Read the model definition and answer for the solid it produces. Units are mm, in the model's axes. Face numbers are marked on the shaded views. Give positions to 0.01 mm unless a question says otherwise; leave off trailing zeros. Write each loop counter-clockwise with the first axis right and the second up, starting at its lowest first coordinate (ties: lowest second). Pieces come first, ordered by that corner, then holes. Notation, with made-up numbers: (26.5, 51.25) -> (85.5, 51.25) arc R10 cw to (85.5, 69.25) -> close; hole circle Ø2 at (81, 3.25). An arc over 180 degrees is marked (long way). Use a Markdown table: item, result.
from build123d import *

# Parameters (mm, degrees)
CROQUIS1_R              = 105
CROQUIS1_R_2            = 95
SALIENTE_EXTRUIR1_DEPTH = 180
CROQUIS2_R              = 101.5
SALIENTE_EXTRUIR2_DEPTH = 20
REDONDEO1_R             = 15


with BuildPart() as part:
    # Croquis1 → Saliente-Extruir1 (new body)
    with BuildSketch(Plane.XY):
        with Locations(Location((0, 0, 0), (0, 0, 180))):
            Circle(CROQUIS1_R)
        with Locations(Location((0, 0, 0), (0, 0, 180))):
            Circle(CROQUIS1_R_2, mode=Mode.SUBTRACT)
    extrude(amount=SALIENTE_EXTRUIR1_DEPTH)

    # Croquis2 → Saliente-Extruir2 (add)
    with BuildSketch(Plane.XY.offset(180)):
        Circle(CROQUIS2_R)
    extrude(amount=-SALIENTE_EXTRUIR2_DEPTH)

    # Redondeo1
    redondeo1_edges = [part.edges().sort_by_distance(p)[0] for p in [
        (105, 0, 180),
    ]]
    fillet(redondeo1_edges, radius=REDONDEO1_R)


solid = part.part
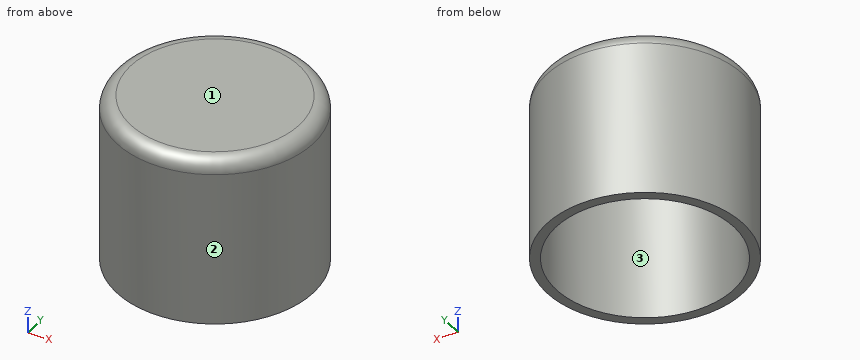
Item 1: For a pull along Y with two mould halves and no side action, classify the marked faces 1, 2 and 3 as +Y half, -Y half, draft (parallel to the pull), parting line (faces both ways), or undercut.
Return value:
| item | result |
|---|---|
| face 1 | draft |
| face 2 | parting line |
| face 3 | undercut |
Item 2: A cutting plane is placed at A-A (x = 0). Give the vertices of the cut face in (y, z), then the cut area to 3 significant figures.
Return value:
| item | result |
|---|---|
| outline | (-105, 0) -> (-95, 0) -> (-95, 160) -> (95, 160) -> (95, 0) -> (105, 0) -> (105, 165) arc R15 ccw to (90, 180) -> (-90, 180) arc R15 ccw to (-105, 165) -> close |
| area | 7,300 mm^2 |
Item 3: A cutting plane is placed at B-B (z = 110). Give the vertices of the cut face in (x, y).
Return value:
| item | result |
|---|---|
| outline | circle Ø210 at (0, 0); hole circle Ø190 at (0, 0) |
Item 4: Straight lines are drawn through the part: line 1 along Y through (x, z) = (0, 97); line 2 along Z through (x, y) = (-28.5, -54); line 3 along X through (y, z) = (-34, 140.5). For each, find the intervals that lie inside material, in ascending order. Write a range as [from, to].
Return value:
| item | result |
|---|---|
| line 1 | [-105, -95], [95, 105] |
| line 2 | [160, 180] |
| line 3 | [-99.34, -88.71], [88.71, 99.34] |
Item 5: Each of these flat-tipped pins is pushed along its axis until it touches: P1, Ø4, axis at x = 76, y = 42.5, coming from the -Z side; P2, Ø8, axis at x = -11, z = 62.5, coming from the +Y side; P3, Ø1, axis at y = 70.5, z = 44, coming from the -X side. Where does it stop, or does it pass through?
Return value:
| item | result |
|---|---|
| P1 | z = 160 |
| P2 | y = 104.77 |
| P3 | x = -78.26 |
